```python
from build123d import *


with BuildPart() as f1:
    # F0 (on Top) → F1 (revolve)
    with BuildSketch(Plane.XY):
        with BuildLine():
            Line((0, 12.7), (0, 25.4))
            ThreePointArc((0, 25.4), (-12.7, 21.9970452561), (-21.9970452561, 12.7))
            Line((-21.9970452561, 12.7), (0, 12.7))
        make_face()
        with BuildLine():
            ThreePointArc((0, -25.4), (17.9605122421, -17.9605122421), (25.4, 0))
            ThreePointArc((25.4, 0), (17.9605122421, 17.9605122421), (0, 25.4))
            Line((0, 25.4), (0, 12.7))
            Line((0, 12.7), (0, 0))
            Line((0, 0), (0, -12.7))
            Line((0, -12.7), (0, -25.4))
        make_face()
        with BuildLine():
            ThreePointArc((-21.9970452561, -12.7), (-12.7, -21.9970452561), (0, -25.4))
            Line((0, -25.4), (0, -12.7))
            Line((0, -12.7), (-21.9970452561, -12.7))
        make_face()
    revolve(axis=Axis((114.3, 14.0205519274, 0), (0, 1, 0)))


solid = f1.part
```
The listing builds one solid part. Answer for the finished solid, in the listing's coordinates (mm). Coordinates: 2 decimals unless noted, no trailing zeros. Write each loop counter-clockwise with the first axis right and the second up, starting at its lowest first coordinate (ties: lowest second). Pieces come first, ordered by that corner, then holes. Notation, with made-up numbers: (73, -29) - (112, -29) arc R19 cw to (112, 6) - close; hole circle Ø2 at (26.5, -27.75). An arc over 180 degrees is marked (long way). Return JSON: item names as keys, results as strings. Group by question number.
1. Given pin 1 (10 mm diameter, centred on y = -19.5, z = 54, fed in from -X); pin 2 (4 mm diameter, centred on y = -1, z = -80.5, fed in from -X); pin 3 (6 mm diameter, centred on x = 205, z = 64, fed in from +Y), each flat-ended and moving along its own axis, determine where each tip first touches the part or whether it passes through.
2. Straight lines are drawn through the part: L1, parallel to Y at x = 204.5, z = 73; L2, parallel to X at y = -7.5, z = 75; L3, parallel to Z at x = 108.5, y = 12. For each, find the intervals that lie inside material, in ascending order.
3. A cutting plane is placed at A-A, the plane y = -6.5. Determine the outline of the cut face in (x, z).
4. A cutting plane is placed at B-B, the plane y = 20. Determine the outline of the cut face in (x, z), plus the area to 3 significant figures.
Ans:
{
 "1": {"pin 1": "x = -10.14", "pin 2": "x = 31.22", "pin 3": "y = 25.4"},
 "2": {"L1": "-25.34 to -12.7, 12.7 to 25.34", "L2": "28.05 to 64.49, 164.11 to 200.55", "L3": "-114.15 to -91.73, 91.73 to 114.15"},
 "3": {"outline": "circle Ø228.6 at (114.3, 0); hole circle Ø179.49 at (114.3, 0)"},
 "4": {"outline": "circle Ø259.92 at (114.3, 0); hole circle Ø197.28 at (114.3, 0)", "area": "22,500 mm²"}
}
